from build123d import *

# Parameters (mm, degrees)
SKETCH1_W           = 10
SKETCH1_H           = 45
SKETCH1_R           = 2.16
BOSS_EXTRUDE1_DEPTH = 5
CUT_EXTRUDE1_DEPTH  = 3.1
BOSS_EXTRUDE2_DEPTH = 10
FILLET1_R           = 2.5


with BuildPart() as part:
    # Sketch1 → Boss-Extrude1 (new body)
    with BuildSketch(Plane(origin=(0, 0, 0), x_dir=(1, 0, 0), z_dir=(0, 1, 0))):
        with Locations((5, 22.5)):
            Rectangle(SKETCH1_W, SKETCH1_H)
        with Locations(Location((5, 37.205, 0), (0, 0, 270))):
            Circle(SKETCH1_R, mode=Mode.SUBTRACT)
        with Locations(Location((5, 7.795, 0), (0, 0, 270))):
            Circle(SKETCH1_R, mode=Mode.SUBTRACT)
    extrude(amount=BOSS_EXTRUDE1_DEPTH)

    # Sketch2 → Cut-Extrude1 (cut)
    with BuildSketch(Plane(origin=(0, 5, 0), x_dir=(1, 0, 0), z_dir=(0, 1, 0))):
        Polygon((5, 32.7016679), (8.9, 34.95333395), (8.9, 39.45666605), (5, 41.7083321), (1.1, 39.45666605), (1.1, 34.95333395), align=None)
        Polygon((5, 12.2983321), (1.1, 10.04666605), (1.1, 5.54333395), (5, 3.2916679), (8.9, 5.54333395), (8.9, 10.04666605), align=None)
    extrude(amount=-CUT_EXTRUDE1_DEPTH, mode=Mode.SUBTRACT)

    # Sketch3 → Boss-Extrude2 (add, through all)
    with BuildSketch(Plane.ZY):
        Polygon((-25, 5), (-25, 11.5), (-40, 11.5), (-40, 9), (-45, 9), (-45, 16.25), (0, 16.25), (0, 9), (-5, 9), (-5, 11.5), (-20, 11.5), (-20, 5), align=None)
    extrude(amount=-BOSS_EXTRUDE2_DEPTH)

    # Fillet1
    fillet1_edges = [part.edges().sort_by_distance(p)[0] for p in [
        (5, 5, -45),
        (5, 5, -20),
        (5, 5, -25),
        (5, 9, -45),
        (5, 9, 0),
        (5, 5, 0),
    ]]
    fillet(fillet1_edges, radius=FILLET1_R)


solid = part.part
The listing builds one solid part. Answer for the finished solid, in the listing's coordinates (mm). A direction names the side the tool comes from. Round coordinates to 2 decimals unless told otherwise and drop trailing zeros. Write each loop counter-clockwise with the first axis right and the second up, starting at its lowest first coordinate (ties: lowest second). Pieces come first, ordered by that corner, then holes. Notation, with made-up numbers: (61.5, -16.5) - (96.5, -16.5) arc R29 ccw to (96.5, 11.5) - close; hole circle Ø7 at (53, -29.5). An arc over 180 degrees is marked (long way). Use a Markdown table: item, result. Add a question column.
1. Consider line 1 (Z direction, x = 5, y = 1.45) (3 decimals); line 2 (Y direction, x = 4.5, z = -30.5); line 3 (Z direction, x = 3.25, y = 4.75). Determine where each line is inside the solid, lowest interval first.
2. A tool of negligible diameter and unlimited length cuts with its end or side. For faces 1 (the face through (5, 9, -41)), 2 (the face through (3.08, 3.47, -40.6)), 3 (the face through (5, 10, -5)), from which of +Z, -Z, +X, -X, +Y, -Y can it reach the whole face along a straight path? Write none if from no direction.
3. The part is cut by section A-A (z = -19). Write down the section's boundary in (x, y).
4. A flat-ended cylindrical pin translates along its axis: P1, Ø5, axis at x = 4, y = 3.5, coming from the -Z side. Find the tip coordinate at first contact, or state that the pin passes through.
5. The part is cut by section B-B (x = 9.5). Write down the section's boundary in (y, z).
6. The part is cut by section D-D (x = 4.5). Give the number of separate pieces and of enclosed holes in the cut face, and give its area (3 significant figures).
7. For a pull along Y with two mould halves and no side action, classify faces 4 (the face through (6.9, 3.5, -33.8)), 5 (the face through (5.07, 9.752, -0.713)), 6 (the face through (5, 16.25, -23)), 7 (the face through (5.095, 0.937, -39.363)) as +Y half, -Y half, draft (parallel to the pull), parting line (faces both ways), or undercut.
8. The part is cut by section C-C (y = 1.5). Write down the section's boundary in (x, z) (3 decimals), and give its area (3 significant figures).
Reported:
| question | item | result |
|---|---|---|
| 1 | line 1 | -45 to -39.365, -35.045 to -9.955, -5.635 to 0 |
| 1 | line 2 | 0 to 5, 11.5 to 16.25 |
| 1 | line 3 | -43.59 to -40.7, -33.71 to -11.29, -4.3 to -1.41 |
| 2 | face 1 | -Z, +X, -X |
| 2 | face 2 | none |
| 2 | face 3 | +X, -X |
| 3 | outline | (0, 0) - (10, 0) - (10, 5.5) - (0, 5.5) - close; (0, 11.5) - (10, 11.5) - (10, 16.25) - (0, 16.25) - close |
| 4 | P1 | z = -45 |
| 5 | outline | (0, -45) - (2.5, -45) arc R2.5 ccw to (5, -42.5) - (5, -27.5) arc R2.5 cw to (7.5, -25) - (11.5, -25) - (11.5, -40) - (9, -40) - (9, -42.5) arc R2.5 ccw to (11.5, -45) - (16.25, -45) - (16.25, 0) - (11.5, 0) arc R2.5 ccw to (9, -2.5) - (9, -5) - (11.5, -5) - (11.5, -20) - (7.5, -20) arc R2.5 cw to (5, -17.5) - (5, -2.5) arc R2.5 ccw to (2.5, 0) - (0, 0) - close |
| 6 | separate pieces | 3 |
| 6 | enclosed holes | 0 |
| 6 | area | 425 mm^2 |
| 7 | face 4 | undercut |
| 7 | face 5 | undercut |
| 7 | face 6 | +Y half |
| 7 | face 7 | draft |
| 8 | outline | (0, -45) - (10, -45) - (10, 0) - (0, 0) - close; hole circle Ø4.32 at (5, -37.205); hole circle Ø4.32 at (5, -7.795) |
| 8 | area | 421 mm^2 |
